Autodesk Inventor part; units mm, degrees
ref_plane "YZ Plane" through (0, 0, 0) normal (1, 0, 0) x (0, 1, 0)
ref_plane "XZ Plane" through (0, 0, 0) normal (0, 1, 0) x (-1, 0, 0)
ref_plane "XY Plane" through (0, 0, 0) normal (0, 0, 1) x (1, 0, 0)
sketch "Sketch1" plane through (0, 0, 0) normal (0, 0, 1) x (1, 0, 0)
  line L0 (0, 0) -> (30, 0)
  line L1 (30, 0) -> (30, 20)
  line L2 (30, 20) -> (0, 20)
  line L3 (0, 20) -> (0, 0)
  dimension "d0" = 30
  dimension "d1" = 20
extrude "Extrusion1" add sketch "Sketch1" along normal blind 50
sketch "Sketch2" plane through (0, 20, 0) normal (0, 1, 0) x (1, 0, 0)
  line L0 (30, 0) -> (0, 0)
  line L1 (0, 0) -> (0, -50)
  line L2 (30, -50) -> (0, -50)
  line L3 (30, 0) -> (30, -50)
  line L4 (7, -50) -> (23, -50)
  line L5 (23, -50) -> (23, -15)
  line L6 (23, -15) -> (7, -15)
  line L7 (7, -15) -> (7, -50)
  point P0 (0, 0)
  dimension "d5" = 7
  dimension "d8" = 15
  dimension "d26" = 7
extrude "Extrusion2" cut sketch "Sketch2" against normal up to next contours L2 L7 L6 L5
sketch "Sketch3" plane through (30, 0, 0) normal (1, 0, 0) x (0, 0, -1)
  line L0 (0, 0) -> (0, 20)
  line L1 (0, 20) -> (-50, 20)
  line L2 (-50, 0) -> (-50, 20)
  line L3 (0, 0) -> (-50, 0)
  circle A0 centre (-40, 10) radius 2.5
  point P0 (0, 0)
  dimension "d11" = 5
  dimension "d12" = 10
  dimension "d13" = 10
extrude "Extrusion3" cut sketch "Sketch3" against normal through all contours A0
sketch "Sketch4" plane through (7, 20, 15) normal (0, 0, 1) x (1, 0, 0)
  line L0 (16, -20) -> (0, -20)
  line L1 (16, 0) -> (16, -20)
  line L2 (0, 0) -> (16, 0)
  line L3 (0, 0) -> (0, -20)
  circle A0 centre (8, -10) radius 5
  line L4 (-7, 0) -> (-7, -20)
  dimension "d16" = 10
  dimension "d17" = 10
  dimension "d29" = 15
extrude "Extrusion4" cut sketch "Sketch4" against normal blind 5 contours A0
sketch "Sketch5" plane through (15, 10, 10) normal (0, 0, 1) x (1, 0, 0)
  circle A0 centre (0, 0) radius 3.175
  line L0 (8, -10) -> (-8, -10)
  line L1 (-8, -10) -> (-8, 10)
  line L2 (-15, 10) -> (-15, -10)
  dimension "d21" = 6.35
  dimension "d22" = 10
  dimension "d30" = 15
extrude "Extrusion5" cut sketch "Sketch5" against normal up to next
fillet "Fillet1" radius 2 1 edges at (7, 10, 15)
fillet "Fillet2" radius 2 1 edges at (23, 10, 15)
properties part number "X_Rail_Belt_Pulley_Connector(2)"
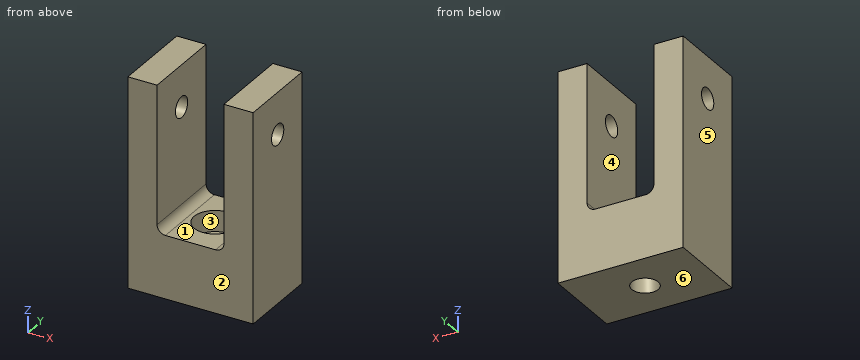
The listing builds one solid part. Answer for the finished solid, in the listing's coordinates (mm). Face numbers are marked on the shaded views. A direction names the side the tool comes from. Coordinates: 2 decimals unless noted, no trailing zeros. Loops run counter-clockwise (first coordinate to the right, second up) from the corner with the lowest first, then second, coordinate; pieces in that order, holes last. Notation, with made-up numbers: M 43.25,64.5 L 93.25,64.5 A37 ccw 93.25,102.5 Z; hole C 64.5,1 d8. An arc over 180 degrees is marked long. Answer in a Markdown table with one row per item.
1) Find section D-D (z = 40). Determine the outline of the cut face in (x, y).
Answers below:
| item | result |
|---|---|
| outline | M 0,0 L 7,0 L 7,7.5 L 0,7.5 Z; M 0,12.5 L 7,12.5 L 7,20 L 0,20 Z; M 23,0 L 30,0 L 30,7.5 L 23,7.5 Z; M 23,12.5 L 30,12.5 L 30,20 L 23,20 Z |
2) Given pin 1 (6 mm diameter, centred on x = 16, y = 12.5, fed in from +Z); pin 2 (6 mm diameter, centred on x = 15, y = 10, fed in from -Z); pin 3 (10 mm diameter, centred on y = 7.5, z = 41.5, fed in from -X), each flat-ended and moving along its own axis, determine where each tip first touches the part or whether it passes through.
Answers below:
| item | result |
|---|---|
| pin 1 | z = 15 |
| pin 2 | through |
| pin 3 | x = 0 |
3) Which of the six approach directions +Z, -Z, +X, -X, +Y, -Y give full straight-line access (tool end or side, diameter ignored) to the marked faces 1, 2 and 3?
Answers below:
| item | result |
|---|---|
| face 1 | +Z, +Y, -Y |
| face 2 | +Z, -Z, +X, -X, -Y |
| face 3 | +Z |
4) Find section A-A (x = 15). Determine the outline of the cut face in (y, z) (3 decimals), then the cut area to 4 significant figures.
Answers below:
| item | result |
|---|---|
| outline | M 0,0 L 6.825,0 L 6.825,10 L 5,10 L 5,15 L 0,15 Z; M 13.175,0 L 20,0 L 20,15 L 15,15 L 15,10 L 13.175,10 Z |
| area | 186.5 mm^2 |
5) Find the intervals of material crossed by probe 1 along X at (y, z) = (4.75, 26.5); probe 2 along Y at (x, z) = (15, 7) (3 decimals); probe 3 along Y at (x, z) = (15, 11.3), in increasing order.
Answers below:
| item | result |
|---|---|
| probe 1 | 0 to 7, 23 to 30 |
| probe 2 | 0 to 6.825, 13.175 to 20 |
| probe 3 | 0 to 5, 15 to 20 |
6) Find section B-B (z = 47). Determine the outline of the cut face in (x, y), then the cut area to 3 significant figures.
Answers below:
| item | result |
|---|---|
| outline | M 0,0 L 7,0 L 7,20 L 0,20 Z; M 23,0 L 30,0 L 30,20 L 23,20 Z |
| area | 280 mm^2 |
7) Find section C-C (y = 10). Determine the outline of the cut face in (x, z) (3 decimals), then the cut area to 3 significant figures.
Answers below:
| item | result |
|---|---|
| outline | M 0,0 L 11.825,0 L 11.825,10 L 10,10 L 10,15 L 9,15 A2 cw 7,17 L 7,37.5 L 0,37.5 Z; M 0,42.5 L 7,42.5 L 7,50 L 0,50 Z; M 18.175,0 L 30,0 L 30,37.5 L 23,37.5 L 23,17 A2 cw 21,15 L 20,15 L 20,10 L 18.175,10 Z; M 23,42.5 L 30,42.5 L 30,50 L 23,50 Z |
| area | 758 mm^2 |
8) Determine the mould class of the marked faces 4, 5 and 6 for opening direction X: released by +X, released by -X, zero draft, split by the parting line, or undercut.
Answers below:
| item | result |
|---|---|
| face 4 | undercut |
| face 5 | released by -X |
| face 6 | zero draft |
